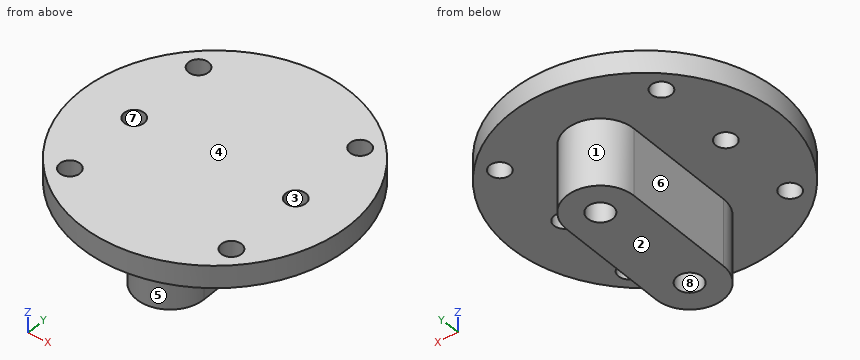
```python
from build123d import *

# Parameters (mm, degrees)
ESQUISSE1_R        = 30
ESQUISSE1_R_2      = 2.25
BOSS_EXTRU_1_DEPTH = 5
ESQUISSE2_R        = 2.8
BOSS_EXTRU_2_DEPTH = 15


with BuildPart() as part:
    # Esquisse1 → Boss.-Extru.1 (new body)
    with BuildSketch(Plane.XY):
        Circle(ESQUISSE1_R)
        with Locations((18, 18)):
            Circle(ESQUISSE1_R_2, mode=Mode.SUBTRACT)
        with Locations((-18, 18)):
            Circle(ESQUISSE1_R_2, mode=Mode.SUBTRACT)
        with Locations((-18, -18)):
            Circle(ESQUISSE1_R_2, mode=Mode.SUBTRACT)
        with Locations((18, -18)):
            Circle(ESQUISSE1_R_2, mode=Mode.SUBTRACT)
        with Locations((18, 0)):
            Circle(ESQUISSE1_R_2, mode=Mode.SUBTRACT)
        with Locations((-18, 0)):
            Circle(ESQUISSE1_R_2, mode=Mode.SUBTRACT)
    extrude(amount=BOSS_EXTRU_1_DEPTH)

    # Esquisse2 → Boss.-Extru.2 (add)
    with BuildSketch(Plane(origin=(0, 0, 0), x_dir=(-1, 0, 0), z_dir=(0, 0, -1))):
        with BuildLine():
            Line((7.5, 12.5), (7.5, -12.5))
            ThreePointArc((7.5, -12.5), (0, -20), (-7.5, -12.5))
            Line((-7.5, -12.5), (-7.5, 12.5))
            ThreePointArc((-7.5, 12.5), (0, 20), (7.5, 12.5))
        make_face()
        with Locations((0, 12.5)):
            Circle(ESQUISSE2_R, mode=Mode.SUBTRACT)
        with Locations((0, -12.5)):
            Circle(ESQUISSE2_R, mode=Mode.SUBTRACT)
    extrude(amount=BOSS_EXTRU_2_DEPTH)


solid = part.part
```
Check sheet for the modelled part. Datum: model origin and axes. Units: mm. Face numbers are marked on the shaded views. A direction names the side the tool comes from. Round coordinates to 2 decimals unless told otherwise and drop trailing zeros. Loops run counter-clockwise (first coordinate to the right, second up) from the corner with the lowest first, then second, coordinate; pieces in that order, holes last. Notation, with made-up numbers: M 43,26 L 56,26 A17 ccw 56,33 Z; hole C -7,-6.75 d8. An arc over 180 degrees is marked long. Answer as a JSON object with one key per item and string values.
1. Access from +Z, -Z, +X, -X, +Y, -Y to the whole of each face (thin tool, end or side, straight path). Record for the marked faces 4, 5, 6, 7 and 8.
Reply:
{"face 4": "+Z, +X, -X, +Y, -Y", "face 5": "-Z, -Y", "face 6": "-Z, -X, +Y, -Y", "face 7": "+Z, -Z", "face 8": "-Z"}
2. Mould release check, pull along Y, two halves, no side actions. Record for the marked faces 1, 2 and 3: pulls with the +Y half, pulls with the -Y half, needs draft (parallel to the pull), parting line crosses it, or undercut.
Reply:
{"face 1": "pulls with the +Y half", "face 2": "needs draft", "face 3": "undercut"}
3. Gauge pin test, flat ends, axial feed: P1, Ø3.5, axis at x = 0, y = -12.5, coming from the -Z side; P2, Ø5, axis at y = -4.5, z = -6.5, coming from the +X side; P3, Ø4, axis at x = 3.5, z = -12.5, coming from the +Y side. Record the tip position at first contact, or that the pin passes through.
Reply:
{"P1": "stops at z = 0", "P2": "stops at x = 7.5", "P3": "stops at y = 19.85"}
4. Section check A-A (x = -18). Record the boundary of the cut face in (y, z), plus the area to 4 significant figures.
Reply:
{"outline": "M -24,0 L -20.25,0 L -20.25,5 L -24,5 Z; M -15.75,0 L -2.25,0 L -2.25,5 L -15.75,5 Z; M 2.25,0 L 15.75,0 L 15.75,5 L 2.25,5 Z; M 20.25,0 L 24,0 L 24,5 L 20.25,5 Z", "area": "172.5 mm²"}
5. Scan lines: line 1 (X direction, y = 18.5, z = 0.25); line 2 (Y direction, x = -18, z = 1.8); line 3 (Y direction, x = -2, z = -8). Record each from-to range of solid material in increasing order.
Reply:
{"line 1": "x = -23.62 to -20.19, -15.81 to 15.81, 20.19 to 23.62", "line 2": "y = -24 to -20.25, -15.75 to -2.25, 2.25 to 15.75, 20.25 to 24", "line 3": "y = -19.73 to -14.46, -10.54 to 10.54, 14.46 to 19.73"}
6. Section check B-B (z = -7.5). Record the boundary of the cut face in (x, y), plus the area to 3 significant figures.
Reply:
{"outline": "M -7.5,-12.5 A7.5 ccw 7.5,-12.5 L 7.5,12.5 A7.5 ccw -7.5,12.5 Z; hole C 0,-12.5 d5.6; hole C 0,12.5 d5.6", "area": "502 mm²"}
7. Section check C-C (y = 19). Record the boundary of the cut face in (x, z), plus the area to 3 significant figures.
Reply:
{"outline": "M -23.22,0 L -20.02,0 L -20.02,5 L -23.22,5 Z; M -15.98,0 L -3.74,0 L -3.74,-15 L 3.74,-15 L 3.74,0 L 15.98,0 L 15.98,5 L -15.98,5 Z; M 20.02,0 L 23.22,0 L 23.22,5 L 20.02,5 Z", "area": "304 mm²"}
8. Section check D-D (x = 0). Record the boundary of the cut face in (y, z).
Reply:
{"outline": "M -30,0 L -20,0 L -20,-15 L -15.3,-15 L -15.3,0 L -9.7,0 L -9.7,-15 L 9.7,-15 L 9.7,0 L 15.3,0 L 15.3,-15 L 20,-15 L 20,0 L 30,0 L 30,5 L -30,5 Z"}
